from build123d import *

# Parameters (mm, degrees)
CYLINDER2051_R               = 1.5
CYLINDER2051_DEPTH           = 50
CYLINDER2051_PLACEMENT_ANGLE = 45
CYLINDER2052_R               = 1.5
CYLINDER2052_DEPTH           = 50
CYLINDER2052_PLACEMENT_ANGLE = 45
CYLINDER2050_R               = 1.5
CYLINDER2050_DEPTH           = 50
CYLINDER2050_PLACEMENT_ANGLE = 45
CYLINDER2049_R               = 1.5
CYLINDER2049_DEPTH           = 50
CYLINDER2049_PLACEMENT_ANGLE = 45
CYLINDER2062_R               = 1.5
CYLINDER2062_DEPTH           = 50
CYLINDER2062_PLACEMENT_ANGLE = 45
CYLINDER2069_R               = 1.5
CYLINDER2069_DEPTH           = 50
CYLINDER2069_PLACEMENT_ANGLE = 45
CYLINDER2085_R               = 3
CYLINDER2085_DEPTH           = 3
CYLINDER2085_PLACEMENT_ANGLE = 45
CYLINDER2081_R               = 3
CYLINDER2081_DEPTH           = 3
CYLINDER2081_PLACEMENT_ANGLE = 45
CYLINDER2091_R               = 3
CYLINDER2091_DEPTH           = 3
CYLINDER2091_PLACEMENT_ANGLE = 45
CYLINDER2067_R               = 3
CYLINDER2067_DEPTH           = 3
CYLINDER2067_PLACEMENT_ANGLE = 45
CYLINDER2080_R               = 3
CYLINDER2080_DEPTH           = 3
CYLINDER2080_PLACEMENT_ANGLE = 45
CYLINDER2088_R               = 3
CYLINDER2088_DEPTH           = 3
CYLINDER2088_PLACEMENT_ANGLE = 45
CYLINDER2061_R               = 8
CYLINDER2061_DEPTH           = 6
BOX802_W                     = 68
BOX802_H                     = 55
BOX802_DEPTH                 = 6


with BuildPart() as obj1:
    # Cylinder2051 → Cylinder2051 (new body)
    with BuildSketch(Plane.XY):
        Circle(CYLINDER2051_R)
    extrude(amount=CYLINDER2051_DEPTH)


with BuildPart() as obj1_1:
    # Cylinder2051 placement: moved
    add(obj1.part.moved(Location((20, 137, 0))).rotate(Axis((20, 137, 0), (0, 0, 1)), CYLINDER2051_PLACEMENT_ANGLE))


with BuildPart() as compound961:
    # Cylinder2052 → Cylinder2052 (new body)
    with BuildSketch(Plane.XY):
        Circle(CYLINDER2052_R)
    extrude(amount=CYLINDER2052_DEPTH)


with BuildPart() as compound961_1:
    # Cylinder2052 placement: moved
    add(compound961.part.moved(Location((-20, 137, 0))).rotate(Axis((-20, 137, 0), (0, 0, 1)), CYLINDER2052_PLACEMENT_ANGLE))

    # Compound961: union obj1
    add(obj1_1.part)


with BuildPart() as obj2:
    # Cylinder2050 → Cylinder2050 (new body)
    with BuildSketch(Plane.XY):
        Circle(CYLINDER2050_R)
    extrude(amount=CYLINDER2050_DEPTH)


with BuildPart() as obj2_1:
    # Cylinder2050 placement: moved
    add(obj2.part.moved(Location((31, 131, 0))).rotate(Axis((31, 131, 0), (0, 0, 1)), CYLINDER2050_PLACEMENT_ANGLE))


with BuildPart() as compound964:
    # Cylinder2049 → Cylinder2049 (new body)
    with BuildSketch(Plane.XY):
        Circle(CYLINDER2049_R)
    extrude(amount=CYLINDER2049_DEPTH)


with BuildPart() as compound964_1:
    # Cylinder2049 placement: moved
    add(compound964.part.moved(Location((-31, 131, 0))).rotate(Axis((-31, 131, 0), (0, 0, 1)), CYLINDER2049_PLACEMENT_ANGLE))

    # Compound964: union obj2
    add(obj2_1.part)


with BuildPart() as obj3:
    # Cylinder2062 → Cylinder2062 (new body)
    with BuildSketch(Plane.XY):
        Circle(CYLINDER2062_R)
    extrude(amount=CYLINDER2062_DEPTH)


with BuildPart() as obj3_1:
    # Cylinder2062 placement: moved
    add(obj3.part.moved(Location((31, 101, 0))).rotate(Axis((31, 101, 0), (0, 0, 1)), CYLINDER2062_PLACEMENT_ANGLE))


with BuildPart() as compound1109:
    # Cylinder2069 → Cylinder2069 (new body)
    with BuildSketch(Plane.XY):
        Circle(CYLINDER2069_R)
    extrude(amount=CYLINDER2069_DEPTH)


with BuildPart() as compound1109_1:
    # Cylinder2069 placement: moved
    add(compound1109.part.moved(Location((-31, 101, 0))).rotate(Axis((-31, 101, 0), (0, 0, 1)), CYLINDER2069_PLACEMENT_ANGLE))

    # Compound1090: union obj3
    add(obj3_1.part)

    # Compound1109: union Compound961, Compound964
    add(compound961_1.part)
    add(compound964_1.part)


with BuildPart() as obj4:
    # Cylinder2085 → Cylinder2085 (new body)
    with BuildSketch(Plane.XY):
        Circle(CYLINDER2085_R)
    extrude(amount=CYLINDER2085_DEPTH)


with BuildPart() as obj4_1:
    # Cylinder2085 placement: moved
    add(obj4.part.moved(Location((31, 131, 0))).rotate(Axis((31, 131, 0), (0, 0, 1)), CYLINDER2085_PLACEMENT_ANGLE))


with BuildPart() as compound1101:
    # Cylinder2081 → Cylinder2081 (new body)
    with BuildSketch(Plane.XY):
        Circle(CYLINDER2081_R)
    extrude(amount=CYLINDER2081_DEPTH)


with BuildPart() as compound1101_1:
    # Cylinder2081 placement: moved
    add(compound1101.part.moved(Location((-31, 131, 0))).rotate(Axis((-31, 131, 0), (0, 0, 1)), CYLINDER2081_PLACEMENT_ANGLE))

    # Compound1101: union obj4
    add(obj4_1.part)


with BuildPart() as compound1101_2:
    # Compound1101 placement: moved
    add(compound1101_1.part.moved(Location((0, 0, 25))))


with BuildPart() as obj5:
    # Cylinder2091 → Cylinder2091 (new body)
    with BuildSketch(Plane.XY):
        Circle(CYLINDER2091_R)
    extrude(amount=CYLINDER2091_DEPTH)


with BuildPart() as obj5_1:
    # Cylinder2091 placement: moved
    add(obj5.part.moved(Location((31, 101, 0))).rotate(Axis((31, 101, 0), (0, 0, 1)), CYLINDER2091_PLACEMENT_ANGLE))


with BuildPart() as compound1103:
    # Cylinder2067 → Cylinder2067 (new body)
    with BuildSketch(Plane.XY):
        Circle(CYLINDER2067_R)
    extrude(amount=CYLINDER2067_DEPTH)


with BuildPart() as compound1103_1:
    # Cylinder2067 placement: moved
    add(compound1103.part.moved(Location((-31, 101, 0))).rotate(Axis((-31, 101, 0), (0, 0, 1)), CYLINDER2067_PLACEMENT_ANGLE))

    # Compound1103: union obj5
    add(obj5_1.part)


with BuildPart() as compound1103_2:
    # Compound1103 placement: moved
    add(compound1103_1.part.moved(Location((0, 0, 21))))


with BuildPart() as obj6:
    # Cylinder2080 → Cylinder2080 (new body)
    with BuildSketch(Plane.XY):
        Circle(CYLINDER2080_R)
    extrude(amount=CYLINDER2080_DEPTH)


with BuildPart() as obj6_1:
    # Cylinder2080 placement: moved
    add(obj6.part.moved(Location((20, 137, 0))).rotate(Axis((20, 137, 0), (0, 0, 1)), CYLINDER2080_PLACEMENT_ANGLE))


with BuildPart() as compound1106:
    # Cylinder2088 → Cylinder2088 (new body)
    with BuildSketch(Plane.XY):
        Circle(CYLINDER2088_R)
    extrude(amount=CYLINDER2088_DEPTH)


with BuildPart() as compound1106_1:
    # Cylinder2088 placement: moved
    add(compound1106.part.moved(Location((-20, 137, 0))).rotate(Axis((-20, 137, 0), (0, 0, 1)), CYLINDER2088_PLACEMENT_ANGLE))

    # Compound1104: union obj6
    add(obj6_1.part)


with BuildPart() as compound1106_2:
    # Compound1104 placement: moved
    add(compound1106_1.part.moved(Location((0, 0, 25))))

    # Compound1106: union Compound1101, Compound1103
    add(compound1101_2.part)
    add(compound1103_2.part)


with BuildPart() as obj7:
    # Cylinder2061 → Cylinder2061 (new body)
    with BuildSketch(Plane(origin=(0, 83, 25), x_dir=(1, 0, 0), z_dir=(0, 0, 1))):
        Circle(CYLINDER2061_R)
    extrude(amount=CYLINDER2061_DEPTH)


with BuildPart() as cut698:
    # Box802 → Box802 (new body)
    with BuildSketch(Plane(origin=(-34, 86, 25), x_dir=(1, 0, 0), z_dir=(0, 0, 1))):
        with Locations((34, 27.5)):
            Rectangle(BOX802_W, BOX802_H)
    extrude(amount=BOX802_DEPTH)

    # Cut692: cut obj7
    add(obj7.part, mode=Mode.SUBTRACT)

    # Cut696: cut Compound1106
    add(compound1106_2.part, mode=Mode.SUBTRACT)

    # Cut698: cut Compound1109
    add(compound1109_1.part, mode=Mode.SUBTRACT)


solid = cut698.part
For this review, take the finished solid that the model builds, in its own axes (mm). A direction names the side the tool comes from. Round coordinates to 2 decimals unless told otherwise and drop trailing zeros. Order: outer loops, then holes, each group sorted by start corner. A loop starts at its lowest first (then second) coordinate and runs counter-clockwise, first axis right, second up. Notation, with made-up numbers: M 0,-16.75 L 40,-16.75 A22 ccw 40,0.25 Z; hole C -19.75,74 d5. An arc over 180 degrees is marked long. Use a Markdown table: item, result. Add a question column.
Item 1: Add section B-B, the plane x = -31. Give the boundary of the cut face in (y, z).
Item 2: Tool access review of faces 1 (the flat face through (33, 131, 28)), 2 (the cylindrical face through (30.804, 99.513, 27.958)): name each direction out of +Z, -Z, +X, -X, +Y, -Y from which nothing blocks a thin tool from reaching the whole face with its end or side.
Item 3: Add section A-A, the plane x = -20. Give the boundary of the cut face in (y, z).
Item 4: Insertion check: pin 1 (2.5 mm diameter, centred on x = 31, y = 101, fed in from +Z); pin 2 (5 mm diameter, centred on x = 31, y = 131, fed in from -Z). Each pin has a flat end and moves straight along its axis. Give the tip position at first contact, or say it passes through.
Item 5: To check wall thickness, follow line 1 along X through (y, z) = (101, 27.9); line 2 along Y through (x, z) = (-31, 28.7); line 3 along Y through (x, z) = (31, 26.65). State the ranges of each line that lie inside material, in increasing order.
Item 6: Add section C-C, the plane y = 101. Give the boundary of the cut face in (x, z).
Geometry results:
| question | item | result |
|---|---|---|
| 1 | outline | M 86,25 L 99.5,25 L 99.5,31 L 86,31 Z; M 102.5,25 L 128,25 L 128,28 L 129.5,28 L 129.5,31 L 102.5,31 Z; M 132.5,28 L 134,28 L 134,25 L 141,25 L 141,31 L 132.5,31 Z |
| 2 | face 1 | -Z |
| 2 | face 2 | +Z, -Z |
| 3 | outline | M 86,25 L 134,25 L 134,28 L 135.5,28 L 135.5,31 L 86,31 Z; M 138.5,28 L 140,28 L 140,25 L 141,25 L 141,31 L 138.5,31 Z |
| 4 | pin 1 | passes through |
| 4 | pin 2 | stops at z = 28 |
| 5 | line 1 | x = -34 to -32.5, -29.5 to 29.5, 32.5 to 34 |
| 5 | line 2 | y = 86 to 99.5, 102.5 to 129.5, 132.5 to 141 |
| 5 | line 3 | y = 86 to 99.5, 102.5 to 128, 134 to 141 |
| 6 | outline | M -34,25 L -32.5,25 L -32.5,31 L -34,31 Z; M -29.5,25 L 29.5,25 L 29.5,31 L -29.5,31 Z; M 32.5,25 L 34,25 L 34,31 L 32.5,31 Z |
